from build123d import *

# Parameters (mm, degrees)
SKETCH1_R               = 17
BOSS_EXTRUDE1_DEPTH     = 3.6
CAVITY1_OUTLINE_R       = 3.15
CAVITY1_DEPTH           = 3.283595969
CAVITY1_START           = 1.183595969
CAVITY1_2_OUTLINE_R     = 3.15
CAVITY1_2_OUTLINE_R_2   = 1.575
CAVITY1_2_DEPTH         = 2.1
SKETCH9_R               = 20
BOSS_EXTRUDE3_DEPTH     = 4
BOSS_EXTRUDE8_DEPTH     = 8
SKETCH2_R               = 0.6
CUT_EXTRUDE1_DEPTH      = 35.23974299
CIRPATTERN1_COUNT       = 6
SKETCH3_R               = 4.596048158
CUT_EXTRUDE2_DEPTH      = 3.283595969
CUT_EXTRUDE3_DEPTH      = 35.23974299
CUT_EXTRUDE3_DEPTH_BACK = 4
SKETCH4_R               = 4
SKETCH6_R               = 1.8
CUT_EXTRUDE4_DEPTH      = 35.23974299


with BuildPart() as part:
    # Sketch1 → Boss-Extrude1 (new body)
    with BuildSketch(Plane.XY):
        Circle(SKETCH1_R)
    extrude(amount=BOSS_EXTRUDE1_DEPTH)

    # Cavity1: read off the stored shape, not the designer's step
    # Cavity1 outline → Cavity1 (cut)
    with BuildSketch(Plane.XY):
        with BuildLine():
            Line((3.9375, 6.819950055), (2.048148228, 15.163776711))
            ThreePointArc((2.048148228, 15.163776711), (0, 16.8), (-2.048148228, 15.163776711))
            Line((-2.048148228, 15.163776711), (-3.9375, 6.819950055))
            Line((-3.9375, 6.819950055), (-12.108141735, 9.355636751))
            ThreePointArc((-12.108141735, 9.355636751), (-14.549226784, 8.4), (-14.156289963, 5.80813996))
            Line((-14.156289963, 5.80813996), (-7.875, 0))
            Line((-7.875, 0), (-14.156289963, -5.80813996))
            ThreePointArc((-14.156289963, -5.80813996), (-14.549226784, -8.4), (-12.108141735, -9.355636751))
            Line((-12.108141735, -9.355636751), (-3.9375, -6.819950055))
            Line((-3.9375, -6.819950055), (-2.048148228, -15.163776711))
            ThreePointArc((-2.048148228, -15.163776711), (0, -16.8), (2.048148228, -15.163776711))
            Line((2.048148228, -15.163776711), (3.9375, -6.819950055))
            Line((3.9375, -6.819950055), (12.108141735, -9.355636751))
            ThreePointArc((12.108141735, -9.355636751), (14.549226784, -8.4), (14.156289963, -5.80813996))
            Line((14.156289963, -5.80813996), (7.875, 0))
            Line((7.875, 0), (14.156289963, 5.80813996))
            ThreePointArc((14.156289963, 5.80813996), (14.549226784, 8.4), (12.108141735, 9.355636751))
            Line((12.108141735, 9.355636751), (3.9375, 6.819950055))
        make_face()
        Circle(CAVITY1_OUTLINE_R, mode=Mode.SUBTRACT)
    extrude(amount=CAVITY1_DEPTH, mode=Mode.SUBTRACT)

    # Cavity1 2 outline → Cavity1 2 (cut)
    with BuildSketch(Plane.XY.offset(CAVITY1_START)):
        Circle(CAVITY1_2_OUTLINE_R)
        Circle(CAVITY1_2_OUTLINE_R_2, mode=Mode.SUBTRACT)
    extrude(amount=CAVITY1_2_DEPTH, mode=Mode.SUBTRACT)

    # Sketch9 → Boss-Extrude3 (add)
    with BuildSketch(Plane.XY.offset(3.6)):
        Circle(SKETCH9_R)
    extrude(amount=BOSS_EXTRUDE3_DEPTH)

    # Sketch12 → Boss-Extrude8 (add)
    with BuildSketch(Plane.XY.offset(7.6)):
        Polygon((0, -23), (19.918584287, -11.5), (19.918584287, 11.5), (0, 23), (-19.918584287, 11.5), (-19.918584287, -11.5), align=None)
    extrude(amount=BOSS_EXTRUDE8_DEPTH)

    # Sketch2 → Cut-Extrude1 (cut, through all)
    with BuildSketch(Plane(origin=(0, 0, 0), x_dir=(-1, 0, 0), z_dir=(0, 0, -1))):
        with Locations((0, 13.5)):
            Circle(SKETCH2_R)
        with Locations((0, 10.5)):
            Circle(SKETCH2_R)
        with Locations((0, 7.5)):
            Circle(SKETCH2_R)
    cut_extrude1 = extrude(amount=-CUT_EXTRUDE1_DEPTH, mode=Mode.SUBTRACT)

    # CirPattern1: Cut-Extrude1 ×6 about axis
    cirpattern1_axis = Axis((0, 0, 0), (0, 0, 1))
    for i in range(1, CIRPATTERN1_COUNT):
        add(cut_extrude1.rotate(cirpattern1_axis, i * 360 / CIRPATTERN1_COUNT), mode=Mode.SUBTRACT)

    # Sketch3 → Cut-Extrude2 (cut)
    with BuildSketch(Plane(origin=(0, 0, 0), x_dir=(-1, 0, 0), z_dir=(0, 0, -1))):
        Circle(SKETCH3_R)
    extrude(amount=-CUT_EXTRUDE2_DEPTH, mode=Mode.SUBTRACT)

    # Sketch4 → Cut-Extrude3 (cut, two sides: drawn at the far end of the back side and taken through both)
    with BuildSketch(Plane.XY.offset(-CUT_EXTRUDE3_DEPTH_BACK)):
        Circle(SKETCH4_R)
    extrude(amount=CUT_EXTRUDE3_DEPTH + CUT_EXTRUDE3_DEPTH_BACK, mode=Mode.SUBTRACT)

    # Sketch6 → Cut-Extrude4 (cut, through all)
    with BuildSketch(Plane(origin=(0, 0, 0), x_dir=(-1, 0, 0), z_dir=(0, 0, -1))):
        with Locations((-7.875, 0)):
            Circle(SKETCH6_R)
        with Locations((7.875, 0)):
            Circle(SKETCH6_R)
    extrude(amount=-CUT_EXTRUDE4_DEPTH, mode=Mode.SUBTRACT)

    # Fillet1
    # a fillet whose section is not a circle: 10 mm, written as the material it takes off along each edge
    with BuildSketch(Plane(origin=(0, 23, -6.83375673), x_dir=(-0.8660254037844386, -0.5000000000000003, 0), z_dir=(0, 0, 1))) as fillet1_piece_1:
        with BuildLine():
            Bezier((5.773502692, 0), (0, 0), (-2.886751346, 5), weights=[1, 2.333333333, 1])
            Line((-2.886751346, 5), (0, 0))
            Line((0, 0), (5.773502692, 0))
        make_face()
    extrude(amount=36.867513459, mode=Mode.SUBTRACT)


solid = part.part
Work out the finished part from the listing and answer in its coordinate system (mm). A direction names the side the tool comes from. Give positions to 0.01 mm unless a question says otherwise; leave off trailing zeros. Order: outer loops, then holes, each group sorted by start corner. A loop starts at its lowest first (then second) coordinate and runs counter-clockwise, first axis right, second up. Notation, with made-up numbers: (65, 76) -> (77, 76) arc R20 ccw to (77, 89) -> close; hole circle Ø9 at (-8, 85). An arc over 180 degrees is marked (long way). Answer as a JSON object with one key per item and string values. Group by question number.
1. Consider line 1 along Z through (x, y) = (-4.5, 6.5); line 2 along Z through (x, y) = (-15.5, 13.5); line 3 along Y through (x, z) = (-2, 7.75). Determine where each line is inside the solid, lowest interval first. Write a range as [from, to].
2. Section B-B on z = 6.5 is taken. Count the separate pieces of the cut face and the enclosed holes in it, plus the area to 3 significant figures.
3. Flat-ended cylindrical pins translate along their axes: pin 1 Ø1.1 at (x, y) = (6.5, 3.75) entering from +Z; pin 2 Ø1.9 at (x, y) = (-11.69, -6.75) entering from -Z; pin 3 Ø6.5 at (y, z) = (3, 11.5) entering from -X; pin 4 Ø4 at (x, y) = (-18, 12.5) entering from -Z. Find the tip coordinate at first contact, or state that the pin passes through.
4. Section A-A on y = 0 is taken. Determine the outline of the cut face in (x, z) (3 decimals).
5. Section D-D on y = 5.25 is taken. Determine the outline of the cut face in (x, z), plus the area to 3 significant figures.
6. A tool of negligible diameter and unlimited length cuts with its end or side. For faces 3 (the flat face through (4.15, -0.12, 15.6)), 4 (the flat face through (-8.08, -8.106, 1.619)), 5 (the flat face through (18, 10, 7.6)), from which of +Z, -Z, +X, -X, +Y, -Y can it reach the whole face along a straight path? Write none if from no direction.
7. The mould has two halves that part along X. Classify faces 1 (the flat face through (3.006, 10.933, 1.619)), 2 (the flat face through (-18, -10, 7.6)): released by +X, released by -X, zero draft, split by the parting line, or undercut.
8. Section C-C on y = -13.5 is taken. Determine the outline of the cut face in (x, z).
Result sheet:
{
 "1": {"line 1": "z = [3.28, 15.6]", "line 2": "z = [7.6, 15.6]", "line 3": "y = [-21.85, -3.46], [3.46, 21.67]"},
 "2": {"separate pieces": "1", "enclosed holes": "21", "area": "1,170 mm^2"},
 "3": {"pin 1": "passes through", "pin 2": "stops at z = 3.28", "pin 3": "stops at x = -19.92", "pin 4": "stops at z = 3.6"},
 "4": {"outline": "(-20, 3.6) -> (-17, 3.6) -> (-17, 0) -> (-9.675, 0) -> (-9.675, 15.6) -> (-19.919, 15.6) -> (-19.919, 7.6) -> (-20, 7.6) -> close; (-6.075, 3.284) -> (-4, 3.284) -> (-4, 15.6) -> (-6.075, 15.6) -> close; (4, 3.284) -> (6.075, 3.284) -> (6.075, 15.6) -> (4, 15.6) -> close; (9.675, 0) -> (17, 0) -> (17, 3.6) -> (20, 3.6) -> (20, 7.6) -> (19.919, 7.6) -> (19.919, 15.6) -> (9.675, 15.6) -> close"},
 "5": {"outline": "(-19.92, 7.6) -> (-19.3, 7.6) -> (-19.3, 3.6) -> (-16.17, 3.6) -> (-16.17, 0) -> (-13.55, 0) -> (-13.55, 3.28) -> (-9.69, 3.28) -> (-9.69, 15.6) -> (-19.92, 15.6) -> close; (-8.49, 3.28) -> (8.49, 3.28) -> (8.49, 15.6) -> (-8.49, 15.6) -> close; (9.69, 3.28) -> (13.55, 3.28) -> (13.55, 0) -> (16.17, 0) -> (16.17, 3.6) -> (19.3, 3.6) -> (19.3, 7.6) -> (19.92, 7.6) -> (19.92, 15.6) -> (9.69, 15.6) -> close", "area": "471 mm^2"},
 "6": {"face 3": "+Z, +X, -X, +Y, -Y", "face 4": "-Z", "face 5": "-Z, +X, +Y"},
 "7": {"face 1": "undercut", "face 2": "zero draft"},
 "8": {"outline": "(-16.45, 7.6) -> (-14.76, 7.6) -> (-14.76, 3.6) -> (-10.33, 3.6) -> (-10.33, 0) -> (-2.42, 0) -> (-2.42, 3.28) -> (-0.6, 3.28) -> (-0.6, 15.6) -> (-16.45, 15.6) -> close; (0.6, 3.28) -> (2.42, 3.28) -> (2.42, 0) -> (10.33, 0) -> (10.33, 3.6) -> (14.76, 3.6) -> (14.76, 7.6) -> (16.45, 7.6) -> (16.45, 15.6) -> (0.6, 15.6) -> close"}
}
